Could you check a few things on this model? Use its own coordinates, in mm. A direction names the side the tool comes from. Round coordinates to 2 decimals unless told otherwise and drop trailing zeros. Write each loop counter-clockwise with the first axis right and the second up, starting at its lowest first coordinate (ties: lowest second). Pieces come first, ordered by that corner, then holes. Notation, with made-up numbers: (54.5, 83.25) -> (58.5, 83.25) arc R23 ccw to (58.5, 98.25) -> close; hole circle Ø9 at (4, 0). An arc over 180 degrees is marked (long way). Answer as CSV lines item,"result". Start each with the question number.
Q1. Imagine slicing it at B-B on x = -15.5. Please give me the cut outline in (y, z), and give its area (3 significant figures).
Q2. If we mould it in two halves opening along Z, with no side actions, what happens to faces 4 (the cylindrical face through (-16.77, 2.5, -3.64)), 5 (the flat face through (-12, -2.032, -6)), 6 (the flat face through (-12, 5.08, -6))? For each: pulls with the +Z half, pulls with the -Z half, needs draft (parallel to the pull), parting line crosses it, or undercut.
Q3. Imagine slicing it at D-D on x = -12.25. Please give me the cut outline in (y, z), and give its area (3 significant figures).
Q4. If I drill on line 1 (Y direction, x = -15.5, z = -13); line 2 (Y direction, x = -8.5, z = -6); line 3 (X direction, y = -0.5, z = -6.5), over which ranges is the centre line in solid material (lowest first)? Write a range as [from, to].
Q5. For faces 1 (the flat face through (-12, -3.81, -10)), 2 (the flat face through (-5.8, 0, -6.4)), 3 (the flat face through (-12, -3, -5.273)), which set-ups out of +Z, -Z, +X, -X, +Y, -Y let a thin tool reach every point of the face, with its end or its side?
Q6. Imagine slicing it at C-C on y = -1. Please give me the cut outline in (x, z).
Q7. Imagine slicing it at A-A on z = -4. Please give me the cut outline in (x, y).
Q8. Will these pins go through, and if not, where does the flat tip stop? pin 1 Ø2 at (y, z) = (-1.5, -5.5) entering from +X; pin 2 Ø2 at (x, y) = (-16.5, -3) entering from -Z; pin 3 Ø5 at (y, z) = (0, -2) entering from +X; pin 4 Ø5 at (y, z) = (-2, -0.5) entering from -X.
from build123d import *

# Parameters (mm, degrees)
SKETCH1_R           = 5.715
BOSS_EXTRUDE1_DEPTH = 5.08
SKETCH2_R           = 9.017
BOSS_EXTRUDE2_DEPTH = 3.81
SKETCH3_W           = 18.688246184
SKETCH3_H           = 2.010717395
CUT_EXTRUDE1_DEPTH  = 1.778


with BuildPart() as part:
    # Sketch1 → Boss-Extrude1 (new body)
    with BuildSketch(Plane(origin=(0, 0, 0), x_dir=(1, 0, 0), z_dir=(0, 1, 0))):
        with Locations(Location((-11.700574837, 6.278703551, 0), (0, 0, 270))):
            Circle(SKETCH1_R)
    extrude(amount=BOSS_EXTRUDE1_DEPTH)

    # Sketch2 → Boss-Extrude2 (add)
    with BuildSketch(Plane.XZ):
        with Locations(Location((-11.700574837, -6.278703551, 0), (0, 0, 90))):
            Circle(SKETCH2_R)
    extrude(amount=BOSS_EXTRUDE2_DEPTH)

    # Sketch3 → Cut-Extrude1 (cut)
    with BuildSketch(Plane.XZ.offset(3.81)):
        with Locations((-11.700574837, -6.278703552)):
            Rectangle(SKETCH3_W, SKETCH3_H)
    extrude(amount=-CUT_EXTRUDE1_DEPTH, mode=Mode.SUBTRACT)


solid = part.part
Checks:
1,outline,"(-3.81, -14.46) -> (0, -14.46) -> (0, -10.55) -> (5.08, -10.55) -> (5.08, -2.01) -> (0, -2.01) -> (0, 1.9) -> (-3.81, 1.9) -> (-3.81, -5.27) -> (-2.03, -5.27) -> (-2.03, -7.28) -> (-3.81, -7.28) -> close"
1,area,"102 mm^2"
2,face 4,"parting line crosses it"
2,face 5,"undercut"
2,face 6,"needs draft"
3,outline,"(-3.81, -15.28) -> (0, -15.28) -> (0, -11.97) -> (5.08, -11.97) -> (5.08, -0.59) -> (0, -0.59) -> (0, 2.72) -> (-3.81, 2.72) -> (-3.81, -5.27) -> (-2.03, -5.27) -> (-2.03, -7.28) -> (-3.81, -7.28) -> close"
3,area,"123 mm^2"
4,line 1,"[-3.81, 0]"
4,line 2,"[-2.03, 5.08]"
4,line 3,"[-20.71, -2.69]"
5,face 1,"+Z, -Z, +X, -X, -Y"
5,face 2,"+Y"
5,face 3,"+X, -X, -Y"
6,outline,"circle Ø18.03 at (-11.7, -6.28)"
7,outline,"(-20.42, -3.81) -> (-2.98, -3.81) -> (-2.98, 0) -> (-6.46, 0) -> (-6.46, 5.08) -> (-16.94, 5.08) -> (-16.94, 0) -> (-20.42, 0) -> close"
8,pin 1,"x = -2.68"
8,pin 2,"z = -14.46"
8,pin 3,"x = -2.86"
8,pin 4,"x = -20.1"
